```python
from build123d import *

# Parameters (mm, degrees)
SKETCH_1_W               = 96.91
SKETCH_1_H               = 120
EXTRUDE_1_DEPTH          = 40.26
CUT_EXTRUDE_1_DEPTH      = 637.874859919
CUT_EXTRUDE_1_DEPTH_BACK = 637.874859919
SKETCH_2_R               = 10
CUT_EXTRUDE_2_DEPTH      = 485.260622689
CUT_EXTRUDE_2_DEPTH_BACK = 20
SKETCH_3_R               = 10
CHAMFER_1_SIZE           = 5
SKETCH_4_R               = 14.438127561
CUT_EXTRUDE_3_DEPTH      = 500


with BuildPart() as part:
    # 草图1 → 凸台-拉伸1 (new body)
    with BuildSketch(Plane.XY.offset(52.065067551)):
        with Locations((-417.804133345, 371.961966114)):
            Rectangle(SKETCH_1_W, SKETCH_1_H)
    extrude(amount=-EXTRUDE_1_DEPTH)

    # 草图2 → 切除-拉伸1 (cut, two sides: drawn at the far end of the back side and taken through both)
    with BuildSketch(Plane.XY.offset(52.065067551).offset(-CUT_EXTRUDE_1_DEPTH_BACK)):
        with Locations((-417.804133345, 371.961966114)):
            Circle(SKETCH_2_R)
        with Locations((-494.338767254, 524.640290491)):
            Circle(SKETCH_2_R)
    extrude(amount=CUT_EXTRUDE_1_DEPTH + CUT_EXTRUDE_1_DEPTH_BACK, mode=Mode.SUBTRACT)

    # 草图3 → 切除-拉伸2 (cut, two sides: drawn at the far end of the back side and taken through both)
    with BuildSketch(Plane(origin=(0, 431.961966114, 0), x_dir=(1, 0, 0), z_dir=(0, 1, 0)).offset(-CUT_EXTRUDE_2_DEPTH_BACK)):
        with Locations(Location((-417.804133345, -31.455067551, 0), (0, 0, 90))):
            Circle(SKETCH_3_R)
    extrude(amount=CUT_EXTRUDE_2_DEPTH + CUT_EXTRUDE_2_DEPTH_BACK, mode=Mode.SUBTRACT)

    # 倒角1
    chamfer_1_edges = [part.edges().sort_by_distance(p)[0] for p in [
        (-369.349133345, 311.961966114, 31.935067551),
        (-369.349133345, 431.961966114, 31.935067551),
        (-466.259133345, 431.961966114, 31.935067551),
        (-466.259133345, 311.961966114, 31.935067551),
    ]]
    chamfer(chamfer_1_edges, length=CHAMFER_1_SIZE)

    # 草图4 → 切除-拉伸3 (cut)
    with BuildSketch(Plane.XY.offset(52.065067551)):
        with Locations((-417.804133345, 371.961966114)):
            Circle(SKETCH_4_R)
    extrude(amount=-CUT_EXTRUDE_3_DEPTH, mode=Mode.SUBTRACT)


solid = part.part
```
Source: CAD feature listing. Evaluate the final solid. Frame: model axes, mm. Coordinates: 2 decimals unless noted, no trailing zeros. Loops run counter-clockwise (first coordinate to the right, second up) from the corner with the lowest first, then second, coordinate; pieces in that order, holes last. Notation, with made-up numbers: M 43.5,-32 L 83.5,-32 A17 cw 83.5,-16 Z; hole C -26.5,19 d7. An arc over 180 degrees is marked long. Use a Markdown table: item, result. Add a question column.
Q1. Section query C-C, the plane z = 26.5. Return loops of the section in (x, y).
Q2. Draft query along X for faces 1 (the flat face through (-371.814, 429.427, 32.217)), 2 (the cylindrical face through (-427.72, 421.82, 32.76)), 3 (the flat face through (-418, 411.962, 32)), 4 (the flat face through (-463.72, 429.5, 32.22)). Return one class per face: pulls with the +X half, pulls with the -X half, needs draft (parallel to the pull), parting line crosses it, or undercut.
Q3. Section query D-D, the plane x = -406.5. Return loops of the section in (y, z), and give its area (3 significant figures).
Q4. Section query A-A, the plane x = -421. Return loops of the section in (y, z).
Q5. Material intervals for L1, parallel to X at y = 379, z = 22; L2, parallel to X at y = 373, z = 38; L3, parallel to Y at x = -404.5, z = 22, sorted ascending.
Q6. Section query B-B, the plane z = 20. Return loops of the section in (x, y).
Q7. First-contact query: pin 1 (16 mm diameter, centred on x = -417.8, z = 31.46, fed in from +Y); pin 2 (6 mm diameter, centred on x = -425, z = 36, fed in from +Y). Flat tips, straight axial feed; report the tip coordinate or a pass-through.
Result:
| question | item | result |
|---|---|---|
| 1 | outline | M -466.26,316.96 L -461.26,311.96 L -374.35,311.96 L -369.35,316.96 L -369.35,426.96 L -374.35,431.96 L -409.12,431.96 L -409.12,411.96 L -426.49,411.96 L -426.49,431.96 L -461.26,431.96 L -466.26,426.96 Z; hole C -417.8,371.96 d28.88 |
| 2 | face 1 | pulls with the +X half |
| 2 | face 2 | undercut |
| 2 | face 3 | undercut |
| 2 | face 4 | pulls with the -X half |
| 3 | outline | M 311.96,11.81 L 362.98,11.81 L 362.98,52.07 L 311.96,52.07 Z; M 380.94,11.81 L 431.96,11.81 L 431.96,52.07 L 380.94,52.07 Z |
| 3 | area | 4,110 mm2 |
| 4 | outline | M 311.96,11.81 L 357.88,11.81 L 357.88,52.07 L 311.96,52.07 Z; M 386.04,11.81 L 431.96,11.81 L 431.96,21.98 L 411.96,21.98 L 411.96,40.93 L 431.96,40.93 L 431.96,52.07 L 386.04,52.07 Z |
| 5 | L1 | x = -466.26 to -430.41, -405.2 to -369.35 |
| 5 | L2 | x = -466.26 to -432.2, -403.4 to -369.35 |
| 5 | L3 | y = 311.96 to 366.35, 377.57 to 431.96 |
| 6 | outline | M -466.26,316.96 L -461.26,311.96 L -374.35,311.96 L -369.35,316.96 L -369.35,426.96 L -374.35,431.96 L -461.26,431.96 L -466.26,426.96 Z; hole C -417.8,371.96 d28.88 |
| 7 | pin 1 | stops at y = 411.96 |
| 7 | pin 2 | stops at y = 431.96 |
